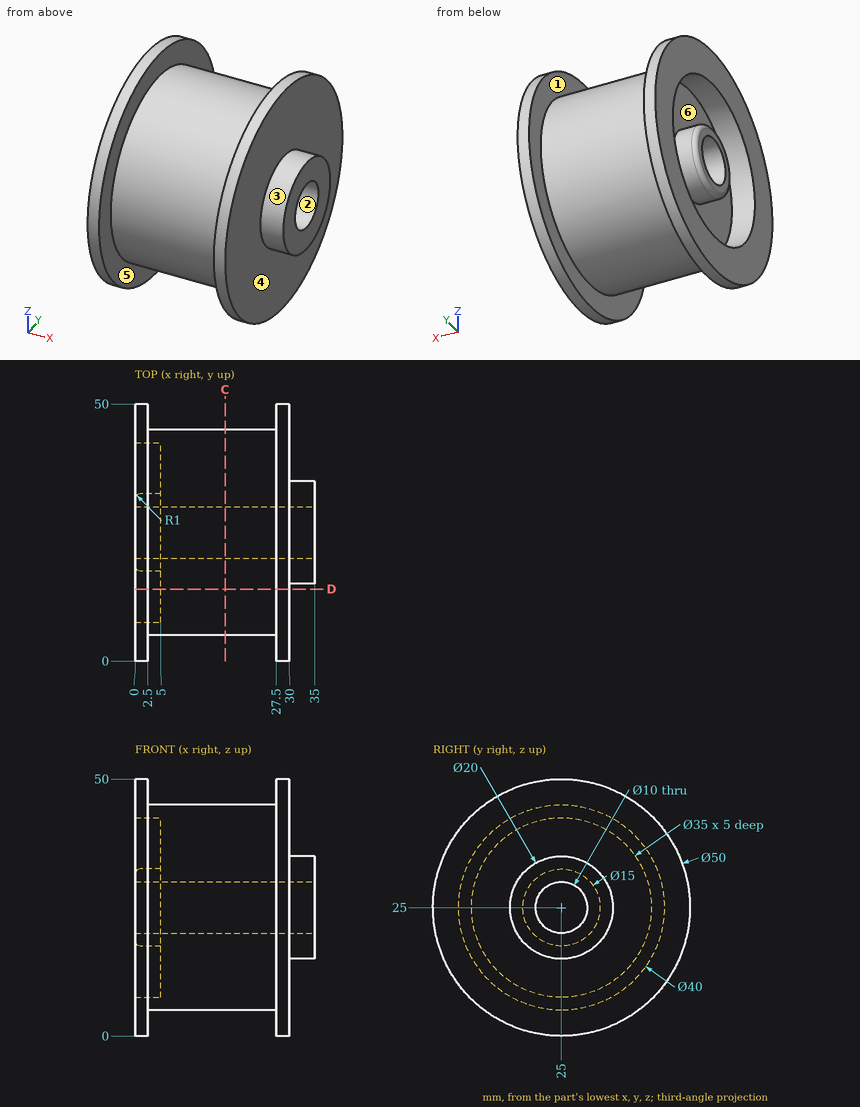
Geometry: see drawing. Coordinates: mm, zero at the bounding-box minimum. A direction names the side the tool comes from. Coordinates: 2 decimals unless noted, no trailing zeros. Loops run counter-clockwise (first coordinate to the right, second up) from the corner with the lowest first, then second, coordinate; pieces in that order, holes last. Notation, with made-up numbers: (68.5, -31.5) - (96.5, -31.5) arc R9 ccw to (96.5, -18.5) - close; hole circle Ø2 at (-26, 5.5). An arc over 180 degrees is marked (long way). Return JSON: item names as keys, results as strings.
Q1. Mould query, pull axis Z, two halves, no side actions, for the marked faces 1, 2 and 3. Classes: released by +Z, released by -Z, zero draft, split by the parting line, or undercut.
Results:
{"face 1": "zero draft", "face 2": "undercut", "face 3": "split by the parting line"}
Q2. Section D-D, the plane y = 14. Return loops of the section in (x, z).
Results:
{"outline": "(0, 2.55) - (2.5, 2.55) - (2.5, 8.3) - (27.5, 8.3) - (27.5, 2.55) - (30, 2.55) - (30, 47.45) - (27.5, 47.45) - (27.5, 41.7) - (2.5, 41.7) - (2.5, 47.45) - (0, 47.45) - (0, 38.61) - (5, 38.61) - (5, 11.39) - (0, 11.39) - close"}
Q3. Material intervals for line 1 along Y through (x, z) = (4, 25); line 2 along Y through (x, z) = (20.5, 25); line 3 along X through (y, z) = (6, 33), sorted ascending.
Results:
{"line 1": "5 to 7.5, 17.5 to 20, 30 to 32.5, 42.5 to 45", "line 2": "5 to 20, 30 to 45", "line 3": "0 to 2.5, 27.5 to 30"}
Q4. Access query for the marked faces 4, 5 and 6. Directions: +Z, -Z, +X, -X, +Y, -Y. A direction counts if a zero-diameter tool reaches every point of the face in a straight line with its end or side. Return the directions, or none.
Results:
{"face 4": "+X", "face 5": "none", "face 6": "-X"}
Q5. Section C-C, the plane x = 17.5. Return loops of the section in (y, z).
Results:
{"outline": "circle Ø40 at (25, 25); hole circle Ø10 at (25, 25)"}
Q6. Contact query for flat-ended pins moving along their axis: P1, Ø5, axis at x = 26, y = 32, coming from the +Z side; P2, Ø5, axis at x = 23.5, z = 23.5, coming from the -Y side; P3, Ø8, axis at x = 27, y = 41, coming from the +Z side; P4, Ø6, axis at y = 25, z = 25, coming from the +X side. Output: stop coordinate, or through.
Results:
{"P1": "z = 49.49", "P2": "y = 5", "P3": "z = 46.91", "P4": "through"}
